The model under review builds one solid part; all positions refer to its coordinate system, in mm. Give positions to 0.01 mm unless a question says otherwise; leave off trailing zeros. Order: outer loops, then holes, each group sorted by start corner. A loop starts at its lowest first (then second) coordinate and runs counter-clockwise, first axis right, second up.
```python
from build123d import *

# Parameters (mm, degrees)
SKETCH_1_W               = 800
SKETCH_1_H               = 1500
SKETCH_1_W_2             = 620
SKETCH_1_H_2             = 1320
EXTRUDE_1_DEPTH          = 18
SKETCH_1_5_W             = 18
SKETCH_1_5_H             = 60
CUT_EXTRUDE_1_DEPTH      = 851.190566873
PATTERN_LINEAR_1_COUNT   = 5
PATTERN_LINEAR_1_PITCH   = 250
MIRROR_1_COPY_1_SKETCH_W = 18
MIRROR_1_COPY_1_SKETCH_H = 60
MIRROR_1_COPY_1_DEPTH    = 851.190566873
MIRROR_1_COPY_2_SKETCH_W = 18
MIRROR_1_COPY_2_SKETCH_H = 60
MIRROR_1_COPY_2_DEPTH    = 851.190566873
MIRROR_1_COPY_3_SKETCH_W = 18
MIRROR_1_COPY_3_SKETCH_H = 60
MIRROR_1_COPY_3_DEPTH    = 851.190566873
MIRROR_1_COPY_4_SKETCH_W = 18
MIRROR_1_COPY_4_SKETCH_H = 60
MIRROR_1_COPY_4_DEPTH    = 851.190566873
SKETCH_1_4_W             = 60
SKETCH_1_4_H             = 18
CUT_EXTRUDE_2_DEPTH      = 851.190566873
PATTERN_LINEAR_2_COUNT   = 3
PATTERN_LINEAR_2_PITCH   = 250
MIRROR_2_COPY_1_SKETCH_W = 60
MIRROR_2_COPY_1_SKETCH_H = 18
MIRROR_2_COPY_1_DEPTH    = 851.190566873
MIRROR_2_COPY_2_SKETCH_W = 60
MIRROR_2_COPY_2_SKETCH_H = 18
MIRROR_2_COPY_2_DEPTH    = 851.190566873
FILLET_1_R               = 25
FILLET_2_R               = 25


with BuildPart() as part:
    # 草图1 → 凸台-拉伸1 (new body)
    with BuildSketch(Plane(origin=(0, 0, 0), x_dir=(1, 0, 0), z_dir=(0, 1, 0))):
        Rectangle(SKETCH_1_W, SKETCH_1_H)
        Rectangle(SKETCH_1_W_2, SKETCH_1_H_2, mode=Mode.SUBTRACT)
    extrude(amount=EXTRUDE_1_DEPTH)

    # 草图1<5> → 切除-拉伸1 (cut, through all)
    with BuildSketch(Plane(origin=(0, 0, 0), x_dir=(1, 0, 0), z_dir=(0, 1, 0))):
        with Locations((-375, -500)):
            Rectangle(SKETCH_1_5_W, SKETCH_1_5_H)
    cut_extrude_1 = extrude(amount=CUT_EXTRUDE_1_DEPTH, mode=Mode.SUBTRACT)

    # 阵列(线性)1: 切除-拉伸1 ×5
    with Locations(*[(0, 0, -i * PATTERN_LINEAR_1_PITCH) for i in range(1, PATTERN_LINEAR_1_COUNT)]):
        add(cut_extrude_1, mode=Mode.SUBTRACT)

    # 镜向1: 切除-拉伸1 across plane
    add(cut_extrude_1.mirror(Plane(origin=(0, 0, 0), x_dir=(0, 0, 1), z_dir=(1, 0, 0))), mode=Mode.SUBTRACT)

    # 镜向1 copy 1 sketch → 镜向1 copy 1 (cut, through all)
    with BuildSketch(Plane(origin=(0, 0, -250), x_dir=(-1, 0, 0), z_dir=(0, 1, 0))):
        with Locations((-375, 500)):
            Rectangle(MIRROR_1_COPY_1_SKETCH_W, MIRROR_1_COPY_1_SKETCH_H)
    extrude(amount=MIRROR_1_COPY_1_DEPTH, mode=Mode.SUBTRACT)

    # 镜向1 copy 2 sketch → 镜向1 copy 2 (cut, through all)
    with BuildSketch(Plane(origin=(0, 0, -500), x_dir=(-1, 0, 0), z_dir=(0, 1, 0))):
        with Locations((-375, 500)):
            Rectangle(MIRROR_1_COPY_2_SKETCH_W, MIRROR_1_COPY_2_SKETCH_H)
    extrude(amount=MIRROR_1_COPY_2_DEPTH, mode=Mode.SUBTRACT)

    # 镜向1 copy 3 sketch → 镜向1 copy 3 (cut, through all)
    with BuildSketch(Plane(origin=(0, 0, -750), x_dir=(-1, 0, 0), z_dir=(0, 1, 0))):
        with Locations((-375, 500)):
            Rectangle(MIRROR_1_COPY_3_SKETCH_W, MIRROR_1_COPY_3_SKETCH_H)
    extrude(amount=MIRROR_1_COPY_3_DEPTH, mode=Mode.SUBTRACT)

    # 镜向1 copy 4 sketch → 镜向1 copy 4 (cut, through all)
    with BuildSketch(Plane(origin=(0, 0, -1000), x_dir=(-1, 0, 0), z_dir=(0, 1, 0))):
        with Locations((-375, 500)):
            Rectangle(MIRROR_1_COPY_4_SKETCH_W, MIRROR_1_COPY_4_SKETCH_H)
    extrude(amount=MIRROR_1_COPY_4_DEPTH, mode=Mode.SUBTRACT)

    # 草图1<4> → 切除-拉伸2 (cut, through all)
    with BuildSketch(Plane(origin=(0, 0, 0), x_dir=(1, 0, 0), z_dir=(0, 1, 0))):
        with Locations((-268, -725)):
            Rectangle(SKETCH_1_4_W, SKETCH_1_4_H)
    cut_extrude_2 = extrude(amount=CUT_EXTRUDE_2_DEPTH, mode=Mode.SUBTRACT)

    # 阵列(线性)2: 切除-拉伸2 ×3
    with Locations(*[(i * PATTERN_LINEAR_2_PITCH, 0, 0) for i in range(1, PATTERN_LINEAR_2_COUNT)]):
        add(cut_extrude_2, mode=Mode.SUBTRACT)

    # 镜向2: 切除-拉伸2 across plane
    add(cut_extrude_2.mirror(Plane.XY), mode=Mode.SUBTRACT)

    # 镜向2 copy 1 sketch → 镜向2 copy 1 (cut, through all)
    with BuildSketch(Plane(origin=(250, 0, 0), x_dir=(1, 0, 0), z_dir=(0, 1, 0))):
        with Locations((-268, 725)):
            Rectangle(MIRROR_2_COPY_1_SKETCH_W, MIRROR_2_COPY_1_SKETCH_H)
    extrude(amount=MIRROR_2_COPY_1_DEPTH, mode=Mode.SUBTRACT)

    # 镜向2 copy 2 sketch → 镜向2 copy 2 (cut, through all)
    with BuildSketch(Plane(origin=(500, 0, 0), x_dir=(1, 0, 0), z_dir=(0, 1, 0))):
        with Locations((-268, 725)):
            Rectangle(MIRROR_2_COPY_2_SKETCH_W, MIRROR_2_COPY_2_SKETCH_H)
    extrude(amount=MIRROR_2_COPY_2_DEPTH, mode=Mode.SUBTRACT)

    # 圆角1
    fillet_1_edges = [part.edges().sort_by_distance(p)[0] for p in [
        (-400, 9, -750),
        (-400, 9, 750),
        (400, 9, 750),
        (400, 9, -750),
    ]]
    fillet(fillet_1_edges, radius=FILLET_1_R)

    # 圆角2
    fillet_2_edges = [part.edges().sort_by_distance(p)[0] for p in [
        (310, 9, -660),
        (-310, 9, -660),
        (-310, 9, 660),
        (310, 9, 660),
    ]]
    fillet(fillet_2_edges, radius=FILLET_2_R)


solid = part.part
```
Item 1: For line 1 (Z direction, x = -45.5, y = 12.75); line 2 (X direction, y = 4.75, z = 513.5); line 3 (Z direction, x = 201.5, y = 10), list the stretches that pass through material, from the lowest coordinate up.
Values found:
line 1: z = -750 to -734, -716 to -660, 660 to 716, 734 to 750
line 2: x = -400 to -384, -366 to -310, 310 to 366, 384 to 400
line 3: z = -750 to -660, 660 to 750
Item 2: Take a section at D-D (y = 5.5). Give the number of separate pieces and of enclosed holes in the cut face, and give its area (3 significant figures).
Values found:
separate pieces: 1
enclosed holes: 17
area: 364,000 mm2
Item 3: Take a section at C-C (z = -145.5). Give the boundary of the cut face in (x, y), and give its area (3 significant figures).
Values found:
outline: (-400, 0) - (-310, 0) - (-310, 18) - (-400, 18) - close; (310, 0) - (400, 0) - (400, 18) - (310, 18) - close
area: 3,240 mm2
Item 4: Take a section at A-A (x = 53.5). Give the boundary of the cut face in (y, z).
Values found:
outline: (0, -750) - (18, -750) - (18, -660) - (0, -660) - close; (0, 660) - (18, 660) - (18, 750) - (0, 750) - close
Item 5: Take a section at B-B (z = 255.5). Give the boundary of the cut face in (x, y).
Values found:
outline: (-400, 0) - (-384, 0) - (-384, 18) - (-400, 18) - close; (-366, 0) - (-310, 0) - (-310, 18) - (-366, 18) - close; (310, 0) - (366, 0) - (366, 18) - (310, 18) - close; (384, 0) - (400, 0) - (400, 18) - (384, 18) - close
